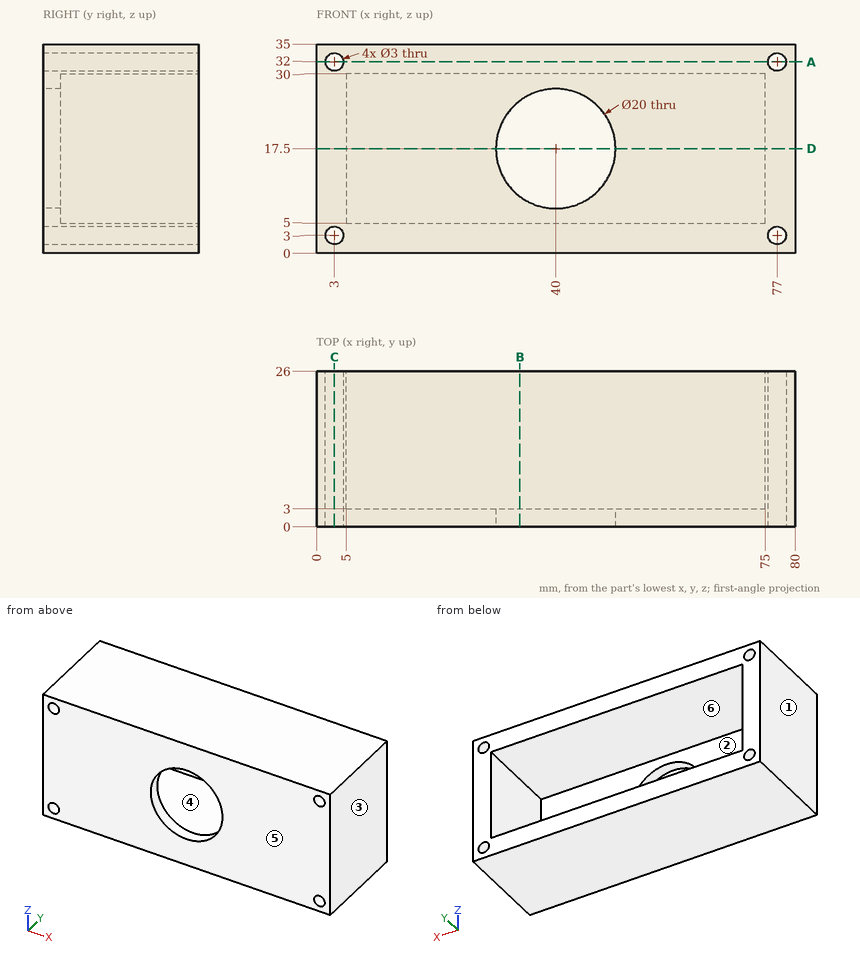
Geometry: see drawing. Coordinates: mm, zero at the bounding-box minimum. A direction names the side the tool comes from. Coordinates: 2 decimals unless noted, no trailing zeros. Loops run counter-clockwise (first coordinate to the right, second up) from the corner with the lowest first, then second, coordinate; pieces in that order, holes last.
Q1. Draft query along X for the marked faces 3, 4, 5 and 6. Return one class per face: +X half, -X half, draft (parallel to the pull), parting line (faces both ways), or undercut.
Q2. Cut plane D-D (z = 17.5). Output: boundary loops of the cut face in (x, y).
Q3. Cut plane B-B (x = 34). Output: boundary loops of the cut face in (y, z), then the cut area to 3 significant figures.
Q4. Contact query for flat-ended pins moving along their axis: pin 1 (1.8 mm diameter, centred on x = 3, z = 32, fed in from +Y); pin 2 (7.5 mm diameter, centred on x = 28.5, z = 12, fed in from +Y). Output: stop coordinate, or through.
Q5. Set-up query: the marked faces 1 and 2. Return all of +Z, -Z, +X, -X, +Y, -Y with unobstructed straight access to the full face (end or side cutting, diameter ignored); none if empty.
Q6. Material intervals for line 1 (Z direction, x = 77, y = 9); line 2 (X direction, y = 9.5, z = 3); line 3 (X direction, y = 15, z = 10), sorted ascending.
Q7. Cut plane A-A (z = 32). Output: boundary loops of the cut face in (x, y), then the cut area to 3 significant figures.
Q8. Cut plane C-C (x = 3). Output: boundary loops of the cut face in (y, z), then the cut area to 3 significant figures.
Working result:
1. face 3: +X half
1. face 4: undercut
1. face 5: draft
1. face 6: undercut
2. outline: (0, 0) - (30, 0) - (30, 3) - (5, 3) - (5, 26) - (0, 26) - close; (50, 0) - (80, 0) - (80, 26) - (75, 26) - (75, 3) - (50, 3) - close
3. outline: (0, 0) - (26, 0) - (26, 5) - (3, 5) - (3, 9.5) - (0, 9.5) - close; (0, 25.5) - (3, 25.5) - (3, 30) - (26, 30) - (26, 35) - (0, 35) - close
3. area: 287 mm2
4. pin 1: passes through
4. pin 2: stops at y = 3
5. face 1: +Z, -Z, -X, +Y, -Y
5. face 2: +Y
6. line 1: z = 0 to 1.5, 4.5 to 30.5, 33.5 to 35
6. line 2: x = 0 to 1.5, 4.5 to 75.5, 78.5 to 80
6. line 3: x = 0 to 5, 75 to 80
7. outline: (0, 0) - (1.5, 0) - (1.5, 26) - (0, 26) - close; (4.5, 0) - (75.5, 0) - (75.5, 26) - (4.5, 26) - close; (78.5, 0) - (80, 0) - (80, 26) - (78.5, 26) - close
7. area: 1,920 mm2
8. outline: (0, 0) - (26, 0) - (26, 1.5) - (0, 1.5) - close; (0, 4.5) - (26, 4.5) - (26, 30.5) - (0, 30.5) - close; (0, 33.5) - (26, 33.5) - (26, 35) - (0, 35) - close
8. area: 754 mm2
